```python
from build123d import *

# Parameters (mm, degrees)
SKETCH1_W           = 500
SKETCH1_H           = 400
BOSS_EXTRUDE1_DEPTH = 6
SKETCH10_W          = 500
SKETCH10_H          = 400
CUT_EXTRUDE4_DEPTH  = 321.21242949


with BuildPart() as part:
    # Sketch1 → Boss-Extrude1 (new body)
    with BuildSketch(Plane(origin=(0, 0, 0), x_dir=(1, 0, 0), z_dir=(0, 1, 0))):
        Rectangle(SKETCH1_W, SKETCH1_H)
    extrude(amount=BOSS_EXTRUDE1_DEPTH)

    # Sketch10 → Cut-Extrude4 (cut, through all)
    with BuildSketch(Plane(origin=(0, 6, 0), x_dir=(1, 0, 0), z_dir=(0, 1, 0))):
        Rectangle(SKETCH10_W, SKETCH10_H)
        with BuildLine():
            Line((-56.474136069, -35.255089794), (-60.116609751, -35.255074272))
            Line((-60.116609751, -35.255074272), (-60.116609751, 5.244926844))
            Line((-60.116609751, 5.244926844), (-66.116640434, 5.244926844))
            Line((-66.116640434, 5.244926844), (-66.116640434, -35.255074272))
            Line((-66.116640434, -35.255074272), (-66.151890674, -35.25504815))
            Line((-66.151890674, -35.25504815), (-97.779213654, -35.254912055))
            Line((-97.779213654, -35.254912055), (-97.779213654, -41.25491222))
            Line((-97.779213654, -41.25491222), (-138.27921477, -41.25491222))
            Line((-138.27921477, -41.25491222), (-138.27921477, -35.254912055))
            Line((-138.27921477, -35.254912055), (-195.884196827, -35.254912055))
            Line((-195.884196827, -35.254912055), (-195.884196827, -11.505116755))
            Line((-195.884196827, -11.505116755), (-195.884196827, -11.5049114))
            Line((-195.884196827, -11.5049114), (-195.884196827, 28.994884362))
            Line((-195.884196827, 28.994884362), (-195.884196827, 28.995089716))
            Line((-195.884196827, 28.995089716), (-195.884196827, 52.745090371))
            Line((-195.884196827, 52.745090371), (-178.779215887, 52.745090371))
            Line((-178.779215887, 52.745090371), (-138.27921477, 52.745090371))
            Line((-138.27921477, 52.745090371), (-138.27921477, 58.745090537))
            Line((-138.27921477, 58.745090537), (-97.779213654, 58.745090537))
            Line((-97.779213654, 58.745090537), (-97.779213654, 52.745090371))
            Line((-97.779213654, 52.745090371), (-57.279212537, 52.745090371))
            Line((-57.279212537, 52.745090371), (-57.279212537, 58.745090537))
            Line((-57.279212537, 58.745090537), (-16.779211421, 58.745090537))
            Line((-16.779211421, 58.745090537), (-16.779211421, 52.745090371))
            Line((-16.779211421, 52.745090371), (23.720789695, 52.745090371))
            Line((23.720789695, 52.745090371), (23.720789695, 58.745090537))
            Line((23.720789695, 58.745090537), (64.220790812, 58.745090537))
            Line((64.220790812, 58.745090537), (64.220790812, 52.745090371))
            Line((64.220790812, 52.745090371), (104.720791928, 52.745090371))
            Line((104.720791928, 52.745090371), (104.720791928, 58.745090537))
            Line((104.720791928, 58.745090537), (145.220793045, 58.745090537))
            Line((145.220793045, 58.745090537), (145.220793045, 52.745090371))
            Line((145.220793045, 52.745090371), (202.825775101, 52.745090371))
            Line((202.825775101, 52.745090371), (202.825775101, 28.995089716))
            Line((202.825775101, 28.995089716), (202.825775101, -11.5049114))
            Line((202.825775101, -11.5049114), (202.825775101, -35.254912055))
            Line((202.825775101, -35.254912055), (185.720794161, -35.254912055))
            Line((185.720794161, -35.254912055), (145.220793045, -35.254912055))
            Line((145.220793045, -35.254912055), (145.220793045, -41.25491222))
            Line((145.220793045, -41.25491222), (104.720791928, -41.25491222))
            Line((104.720791928, -41.25491222), (104.720791928, -35.254912055))
            Line((104.720791928, -35.254912055), (72.732455527, -35.254912055))
            add(Edge.make_bspline(
                [(72.732455674, 5.244926844), (72.732455674, -35.255074272), (72.732455527, -35.254912055)],
                knots=[11, 11, 11, 12, 12, 12], degree=2))
            Line((72.732455674, 5.244926844), (66.732424991, 5.244926844))
            add(Edge.make_bspline(
                [(66.732427246, -35.254912055), (66.732424991, -35.255074272), (66.732424991, 5.244926844)],
                knots=[9, 9, 9, 10, 10, 10], degree=2))
            Line((66.732427246, -35.254912055), (64.220790812, -35.254912055))
            Line((64.220790812, -35.254912055), (64.220790812, -41.25491222))
            Line((64.220790812, -41.25491222), (23.720789695, -41.25491222))
            Line((23.720789695, -41.25491222), (23.720789695, -35.254912055))
            Line((23.720789695, -35.254912055), (-16.779211421, -35.254912055))
            Line((-16.779211421, -35.254912055), (-16.779211421, -41.25491222))
            Line((-16.779211421, -41.25491222), (-56.474136069, -41.25508996))
            Line((-56.474136069, -41.25508996), (-56.474136069, -35.255089794))
        make_face(mode=Mode.SUBTRACT)
    extrude(amount=-CUT_EXTRUDE4_DEPTH, mode=Mode.SUBTRACT)


solid = part.part
```
Source: CAD feature listing. Evaluate the final solid. Frame: model axes, mm. Coordinates: 2 decimals unless noted, no trailing zeros. Answer as a JSON object with one key per item and string values.
1. Cut plane A-A on z = 21. State how many separate pieces and enclosed holes the cut face has, plus the area to 3 significant figures.
Evaluation:
{"separate pieces": "3", "enclosed holes": "0", "area": "2,320 mm^2"}
2. Contact query for flat-ended pins moving along their axis: P1, Ø3, axis at x = -78, y = 2, coming from the -Z side; P2, Ø1.8, axis at y = 3.5, z = -56, coming from the +X side; P3, Ø1.8, axis at y = 2.5, z = 38, coming from the -X side. Output: stop coordinate, or through.
Evaluation:
{"P1": "z = -52.75", "P2": "x = 145.22", "P3": "x = -138.28"}
3. Ray query, L1, parallel to X at y = 3.5, z = -4; L2, parallel to Z at x = 178.5, y = 1.75; L3, parallel to Z at x = 68, y = 4.5. Return the intervals inside material, ascending.
Evaluation:
{"L1": "-195.88 to -66.12, -60.12 to 66.73, 72.73 to 202.83", "L2": "-52.75 to 35.25", "L3": "-52.75 to -5.24"}
